Read the model definition and answer for the solid it produces. Units are mm, in the model's axes. Face numbers are marked on the shaded views. A direction names the side the tool comes from. Coordinates: 2 decimals unless noted, no trailing zeros. Order: outer loops, then holes, each group sorted by start corner. A loop starts at its lowest first (then second) coordinate and runs counter-clockwise, first axis right, second up. Notation, with made-up numbers: M 70.25,46.5 L 111.25,46.5 A10 cw 111.25,53.5 Z; hole C -11.5,78.25 d4. An arc over 180 degrees is marked long. Use a Markdown table: item, result. Add a question column.
1) The mould has two halves that part along X. Classify the marked faces 1, 2 and 3: released by +X, released by -X, zero draft, split by the parting line, or undercut.
2) Find section C-C on y = 55. Write down the section's boundary in (x, z) (1 decimal), plus the area to 3 significant figures.
3) Find section A-A on y = 24. Write down the section's boundary in (x, z) (3 decimals), plus the area to 3 significant figures.
4) Find the intervals of material crossed by probe 1 along Y at (x, z) = (0, 1.7); probe 2 along Z at (x, y) = (-18, 4.5) (3 decimals); probe 3 along Y at (x, z) = (11, -7.5) (3 decimals), in increasing order. Write a range as [from, to].
5) Find section B-B on z = -4.25. Write down the section's boundary in (x, y) (3 decimals).
6) Each of these flat-tipped pins is pushed along its axis until it touches: pin 1 Ø2.5 at (x, y) = (0, 62.22) entering from -Z; pin 2 Ø1 at (y, z) = (57.5, 2) entering from -X; pin 3 Ø1 at (x, z) = (-6, -2.5) entering from -Y; pin 4 Ø1.5 at (y, z) = (-2, -1.5) entering from -X. Where does it stop, or does it pass through?
7) For the marked faces 4, 5, 6 and 7, determine the directions among +Z, -Z, +X, -X, +Y, -Y from which every point of the face is accessible in a straight line to the end or side of a thin tool.
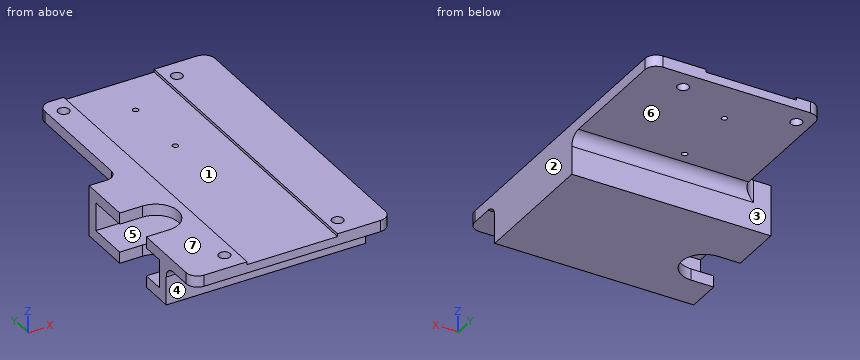
from build123d import *

# Parameters (mm, degrees)
F0_R      = 0.8001
F1_DEPTH  = 3.175
F2_W      = 55.88
F2_H      = 36.83
F3_DEPTH  = 11.1252
F5_DEPTH  = 14.3012
F6_W      = 30.48
F6_H      = 7.9502
F7_DEPTH  = 52.705
F8_W      = 55.88
F8_H      = 3.175
F9_DEPTH  = 12.7
F10_R     = 3.175
F11_R     = 1.5875
F12_DEPTH = 14.3012
F13_W     = 25.4
F13_H     = 1.6002
F14_DEPTH = 87.631


with BuildPart() as f1:
    # F0 (on Top) → F1 (new body)
    with BuildSketch(Plane.XY):
        Polygon((-27.94, 0), (27.94, 0), (27.94, 74.93), (-19.8755, 74.93), (-19.8755, 36.83), (-27.94, 36.83), align=None)
        with Locations((0, 43.1927)):
            Circle(F0_R, mode=Mode.SUBTRACT)
        with Locations((0, 62.2173)):
            Circle(F0_R, mode=Mode.SUBTRACT)
    extrude(amount=F1_DEPTH)

    # F2 (on face) → F3 (join)
    with BuildSketch(Plane(origin=(0, 0, 0), x_dir=(1, 0, 0), z_dir=(0, 0, -1))):
        with Locations((0, -18.415)):
            Rectangle(F2_W, F2_H)
    extrude(amount=F3_DEPTH)

    # F4 (on face) → F5 (cut, through all)
    with BuildSketch(Plane(origin=(0, 0, -11.1252), x_dir=(1, 0, 0), z_dir=(0, 0, -1))):
        with BuildLine():
            Line((-27.94, -9.525), (-27.94, -22.225))
            Line((-27.94, -22.225), (-21.59, -22.225))
            ThreePointArc((-21.59, -22.225), (-15.24, -15.875), (-21.59, -9.525))
            Line((-21.59, -9.525), (-27.94, -9.525))
        make_face()
    extrude(amount=-F5_DEPTH, mode=Mode.SUBTRACT)

    # F6 (on face) → F7 (cut)
    with BuildSketch(Plane(origin=(-27.94, 0, 0), x_dir=(0, -1, 0), z_dir=(-1, 0, 0))):
        with Locations((-18.415, -3.9751)):
            Rectangle(F6_W, F6_H)
    extrude(amount=-F7_DEPTH, mode=Mode.SUBTRACT)

    # F8 (on face) → F9 (join)
    with BuildSketch(Plane.XZ):
        with Locations((0, 1.5875)):
            Rectangle(F8_W, F8_H)
    extrude(amount=F9_DEPTH)

    # F10
    f10_edges = [f1.edges().sort_by_distance(p)[0] for p in [
        (4.03225, 36.83, 0),
        (-19.8755, 36.83, 1.5875),
        (-19.8755, 74.93, 1.5875),
        (27.94, 74.93, 1.5875),
        (0, 0, 0),
        (-27.94, -12.7, 1.5875),
        (27.94, -12.7, 1.5875),
    ]]
    fillet(f10_edges, radius=F10_R)

    # F11 (on face) → F12 (cut, through all)
    with BuildSketch(Plane.XY.offset(3.175)):
        with Locations((-15.8877, 69.5325)):
            Circle(F11_R)
        with Locations((15.8877, 69.5325)):
            Circle(F11_R)
        with Locations((-15.8877, -7.3025)):
            Circle(F11_R)
        with Locations((15.8877, -7.3025)):
            Circle(F11_R)
    extrude(amount=-F12_DEPTH, mode=Mode.SUBTRACT)

    # F13 (on face) → F14 (cut, through all)
    with BuildSketch(Plane.XZ.offset(12.7)):
        with Locations((0, 3.175)):
            Rectangle(F13_W, F13_H)
    extrude(amount=-F14_DEPTH, mode=Mode.SUBTRACT)


solid = f1.part
Check result:
| question | item | result |
|---|---|---|
| 1 | face 1 | undercut |
| 1 | face 2 | released by +X |
| 1 | face 3 | zero draft |
| 2 | outline | M -19.9,0 L 27.9,0 L 27.9,3.2 L 12.7,3.2 L 12.7,2.4 L -12.7,2.4 L -12.7,3.2 L -19.9,3.2 Z |
| 2 | area | 131 mm2 |
| 3 | outline | M -27.94,-11.125 L 27.94,-11.125 L 27.94,3.175 L 12.7,3.175 L 12.7,2.375 L -12.7,2.375 L -12.7,3.175 L -27.94,3.175 L -27.94,0 L 24.765,0 L 24.765,-7.95 L -27.94,-7.95 Z |
| 3 | area | 360 mm2 |
| 4 | probe 1 | y = [-12.7, 42.39], [43.99, 61.42], [63.02, 74.93] |
| 4 | probe 2 | z = [-11.125, -7.95], [0, 3.175] |
| 4 | probe 3 | y = [0, 3.175], [33.655, 36.83] |
| 5 | outline | M -27.94,0 L 27.94,0 L 27.94,36.83 L -27.94,36.83 L -27.94,33.655 L 24.765,33.655 L 24.765,3.175 L -27.94,3.175 Z |
| 6 | pin 1 | stops at z = 0 |
| 6 | pin 2 | stops at x = -19.88 |
| 6 | pin 3 | stops at y = -0.23 |
| 6 | pin 4 | passes through |
| 7 | face 4 | -Z, +X, -X, -Y |
| 7 | face 5 | -X |
| 7 | face 6 | -Z, +X, -X, +Y |
| 7 | face 7 | +Z, +X, -X, +Y, -Y |
